Autodesk Inventor part; units mm, degrees
ref_plane "YZ Plane" through (0, 0, 0) normal (1, 0, 0) x (0, 1, 0)
ref_plane "XZ Plane" through (0, 0, 0) normal (0, 1, 0) x (-1, 0, 0)
ref_plane "XY Plane" through (0, 0, 0) normal (0, 0, 1) x (1, 0, 0)
sketch "Sketch1" plane through (0, 0, 0) normal (0, 1, 0) x (-1, 0, 0)
  circle A0 centre (0, 0) radius 1.5
  dimension "d0" = 3
extrude "Extrusion1" add sketch "Sketch1" along normal blind 10
sketch "Sketch2" plane through (0, 10, 0) normal (0, 1, 0) x (1, 0, 0)
  circle A0 centre (0, 0) radius 2.5
  dimension "d3" = 5
extrude "Extrusion2" add sketch "Sketch2" along normal blind 2
fillet "Fillet1" radius 1.7 1 edges at (-2.5, 12, 0)
chamfer "Chamfer1" distance 0.3 angle 45 1 edges at (1.5, 0, 0)
thread "Thread1"
sketch "Sketch3" plane through (0, 12, 0) normal (0, 1, 0) x (1, 0, 0)
  line L0 (0.5, -2.5) -> (0.5, 2.5)
  line L1 (0.5, 2.5) -> (-0.5, 2.5)
  line L2 (-0.5, 2.5) -> (-0.5, -2.5)
  line L3 (-0.5, -2.5) -> (0.5, -2.5)
  line L4 (0.5, -2.5) -> (-0.5, 2.5) construction
  line L5 (0.5, 2.5) -> (-0.5, -2.5) construction
  line L6 (1.5, -0.5) -> (-1.5, -0.5)
  line L7 (-1.5, -0.5) -> (-1.5, 0.5)
  line L8 (-1.5, 0.5) -> (1.5, 0.5)
  line L9 (1.5, 0.5) -> (1.5, -0.5)
  circle A0 centre (0, 0) radius 2.5
  line L10 (1.5, -0.5) -> (-1.5, 0.5) construction
  line L11 (-1.5, -0.5) -> (1.5, 0.5) construction
  dimension "d12" = 1
  dimension "d13" = 3
  dimension "d14" = 1
extrude "Extrusion3" cut sketch "Sketch3" against normal blind 0.7 contours L3 A0 L0 | A0 L2 L6 L0 | L3 L2 A0 | L6 L2 L8 L0 | L0 L8 L9 L6 | L8 L2 A0 L0 | L6 L7 L8 L2 | A0 L1 L0 | L2 L1 A0
properties part number "M3x10 Screw Nylon" material "Nylon 6"
Source: CAD feature listing. Evaluate the final solid. Frame: model axes, mm. Coordinates: 2 decimals unless noted, no trailing zeros. Write each loop counter-clockwise with the first axis right and the second up, starting at its lowest first coordinate (ties: lowest second). Pieces come first, ordered by that corner, then holes. Notation, with made-up numbers: (71, 71.5) -> (92, 71.5) arc R8 ccw to (92, 79.5) -> close; hole circle Ø8 at (15, -25.75). An arc over 180 degrees is marked (long way). Return JSON: item names as keys, results as strings. Group by question number.
1) Contact query for flat-ended pins moving along their axis: P1, Ø0.8, axis at y = 11.5, z = -1.5, coming from the +X side; P2, Ø0.6, axis at y = 11.5, z = 1.5, coming from the +X side; P3, Ø0.8, axis at x = 1, y = 11.5, coming from the -Z side. Output: stop coordinate, or through.
2) Mould query, pull axis Z, two halves, no side actions, for faces 1 (the face through (-0.54, 10.15, -2.44)), 2 (the face through (0, 11.3, 0)), 3 (the face through (0, 0, 0)). Classes: +Z half, -Z half, draft (parallel to the pull), parting line (faces both ways), or undercut.
3) Ray query, line 1 along X through (y, z) = (0.5, 0.05); line 2 along Y through (x, z) = (-0.1, 1). Return the intervals inside material, ascending.
4) Section query A-A, the plane y = 2.5. Return loops of the section in (x, z), plus the area to 3 significant figures.
From the geometry:
{
 "1": {"P1": "x = 1.87", "P2": "x = 1.76", "P3": "z = -2.12"},
 "2": {"face 1": "parting line", "face 2": "undercut", "face 3": "draft"},
 "3": {"line 1": "-1.5 to 1.5", "line 2": "0 to 11.3"},
 "4": {"outline": "circle Ø3 at (0, 0)", "area": "7.07 mm²"}
}
